Geometry: final body of the model. Coordinates: model frame, mm. A direction names the side the tool comes from. Round coordinates to 2 decimals unless told otherwise and drop trailing zeros. Loops run counter-clockwise (first coordinate to the right, second up) from the corner with the lowest first, then second, coordinate; pieces in that order, holes last. Notation, with made-up numbers: (-27.75, 42) -> (-20.75, 42) arc R26 ccw to (-20.75, 66) -> close; hole circle Ø9 at (37.25, 18). An arc over 180 degrees is marked (long way). Answer in a Markdown table with one row per item.
```python
from build123d import *

# Parameters (mm, degrees)
F0_W     = 19.05
F0_H     = 450.85
F1_DEPTH = 463.55
F2_DEPTH = 19.05


with BuildPart() as f1:
    # F0 (on Top) → F1 (new body)
    with BuildSketch(Plane.XY):
        with Locations((9.525, 263.525)):
            Rectangle(F0_W, F0_H)
        Polygon((0, 508), (0, 488.95), (19.05, 488.95), (844.55, 488.95), (863.6, 488.95), (863.6, 508), align=None)
        with Locations((854.075, 263.525)):
            Rectangle(F0_W, F0_H)
    extrude(amount=F1_DEPTH)

    # F0 (on Top) → F2 (join)
    with BuildSketch(Plane.XY):
        Polygon((0, 38.1), (0, 0), (863.6, 0), (863.6, 38.1), (844.55, 38.1), (844.55, 488.95), (19.05, 488.95), (19.05, 38.1), align=None)
    extrude(amount=F2_DEPTH)


solid = f1.part
```
Item 1: Section query C-C, the plane x = 371.5. Output: boundary loops of the cut face in (y, z), and give its area (3 significant figures).
Ans:
| item | result |
|---|---|
| outline | (0, 0) -> (508, 0) -> (508, 463.55) -> (488.95, 463.55) -> (488.95, 19.05) -> (0, 19.05) -> close |
| area | 18,100 mm2 |
Item 2: First-contact query: P1, Ø21, axis at x = 13.5, z = 136.5, coming from the -Y side; P2, Ø12, axis at x = 380, y = 394.5, coming from the +Z side; P3, Ø6, axis at x = 554.5, y = 302.5, coming from the -Z side. Flat tips, straight axial feed; report the tip coordinate or a pass-through.
Ans:
| item | result |
|---|---|
| P1 | y = 38.1 |
| P2 | z = 19.05 |
| P3 | z = 0 |
Item 3: Section query B-B, the plane y = 336. Output: boundary loops of the cut face in (x, z), and give its area (3 significant figures).
Ans:
| item | result |
|---|---|
| outline | (0, 0) -> (863.6, 0) -> (863.6, 463.55) -> (844.55, 463.55) -> (844.55, 19.05) -> (19.05, 19.05) -> (19.05, 463.55) -> (0, 463.55) -> close |
| area | 33,400 mm2 |
Item 4: Section query A-A, the plane z = 261. Output: boundary loops of the cut face in (x, y).
Ans:
| item | result |
|---|---|
| outline | (0, 38.1) -> (19.05, 38.1) -> (19.05, 488.95) -> (844.55, 488.95) -> (844.55, 38.1) -> (863.6, 38.1) -> (863.6, 508) -> (0, 508) -> close |
Item 5: Mould query, pull axis X, two halves, no side actions, for faces 1 (the flat face through (854, 38.1, 238)), 2 (the flat face through (863.6, 250, 229)), 3 (the flat face through (426, 488.95, 238)), 4 (the flat face through (19.05, 260, 238)). Classes: released by +X, released by -X, zero draft, split by the parting line, or undercut.
Ans:
| item | result |
|---|---|
| face 1 | zero draft |
| face 2 | released by +X |
| face 3 | undercut |
| face 4 | undercut |
Item 6: Set-up query: faces 5 (the flat face through (844.55, 260, 238)), 6 (the flat face through (9, 38.1, 238)), 7 (the flat face through (426, 0, 9)). Return all of +Z, -Z, +X, -X, +Y, -Y with unobstructed straight access to the full face (end or side cutting, diameter ignored); none if empty.
Ans:
| item | result |
|---|---|
| face 5 | +Z, -Y |
| face 6 | +Z, +X, -X, -Y |
| face 7 | +Z, -Z, +X, -X, -Y |
Item 7: Ray query, L1, parallel to X at y = 398.5, z = 26; L2, parallel to Y at x = 484, z = 242.5; L3, parallel to Z at x = 773, y = 481. Return the intervals inside material, ascending.
Ans:
| item | result |
|---|---|
| L1 | 0 to 19.05, 844.55 to 863.6 |
| L2 | 488.95 to 508 |
| L3 | 0 to 19.05 |
